Design review of the part built by this model. Coordinates are the model's own, in mm. Coordinates: 2 decimals unless noted, no trailing zeros. Write each loop counter-clockwise with the first axis right and the second up, starting at its lowest first coordinate (ties: lowest second). Pieces come first, ordered by that corner, then holes. Notation, with made-up numbers: (-2.75, 87.25) - (22.25, 87.25) arc R16 cw to (22.25, 93.25) - close; hole circle Ø2 at (-14.75, 70.25). An arc over 180 degrees is marked (long way). Use a Markdown table: item, result.
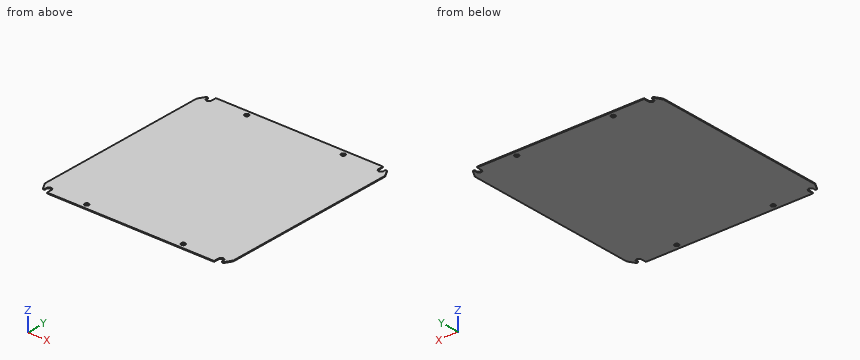
Autodesk Inventor part; units mm, degrees
ref_plane "DPF11_XY" through (224.5, 222.5, 0) normal (0, 0, 1) x (1, 0, 0)
ref_plane "DPF11_YZ" through (224.5, 222.5, 0) normal (1, 0, 0) x (0, 1, 0)
ref_plane "DPF11_ZX" through (224.5, 222.5, 0) normal (0, 1, 0) x (0, 0, 1)
sketch "Skizze_2" plane through (0, 0, 0) normal (0, 0, 1) x (1, 0, 0)
  line L0 (-224.5, 433.5455) -> (-224.5, 11.4545)
  line L1 (-224.5, 11.4545) -> (-215, -5)
  line L2 (-215, -5) -> (-211, -5)
  line L3 (-211, -5) -> (-211, 0)
  arc A0 (-199, 0) -> (-211, 0) centre (-205, 0) ccw
  line L4 (-199, 0) -> (-199, -12.5)
  line L5 (-199, -12.5) -> (199, -12.5)
  line L6 (199, -12.5) -> (199, 0)
  arc A1 (211, 0) -> (199, 0) centre (205, 0) ccw
  line L7 (211, 0) -> (211, -5)
  line L8 (211, -5) -> (215, -5)
  line L9 (215, -5) -> (224.5, 11.4545)
  line L10 (224.5, 11.4545) -> (224.5, 433.5455)
  line L11 (224.5, 433.5455) -> (215, 450)
  line L12 (215, 450) -> (211, 450)
  line L13 (211, 450) -> (211, 445)
  arc A2 (199, 445) -> (211, 445) centre (205, 445) ccw
  line L14 (199, 445) -> (199, 457.5)
  line L15 (199, 457.5) -> (-199, 457.5)
  line L16 (-199, 457.5) -> (-199, 445)
  arc A3 (-211, 445) -> (-199, 445) centre (-205, 445) ccw
  line L17 (-211, 445) -> (-211, 450)
  line L18 (-211, 450) -> (-215, 450)
  line L19 (-215, 450) -> (-224.5, 433.5455)
  circle A4 centre (115, 445) radius 5
  circle A5 centre (115, 0) radius 5
  circle A6 centre (-115, 445) radius 5
  circle A7 centre (-115, 0) radius 5
extrude "Extrusion1" add sketch "Skizze_2" against normal blind 2
ref_plane "DPF11_XY" through (224.5, 222.5, 0) normal (0, 0, 1) x (1, 0, 0)
ref_plane "DPF11_YZ" through (224.5, 222.5, 0) normal (1, 0, 0) x (0, 1, 0)
ref_plane "DPF11_ZX" through (224.5, 222.5, 0) normal (0, 1, 0) x (0, 0, 1)
ref_plane "DPF12_XY" through (-224.5, 222.5, 0) normal (0, 0, 1) x (1, 0, 0)
ref_plane "DPF12_YZ" through (-224.5, 222.5, 0) normal (1, 0, 0) x (0, 1, 0)
ref_plane "DPF12_ZX" through (-224.5, 222.5, 0) normal (0, 1, 0) x (0, 0, 1)
ref_plane "DPF21_XY" through (205, 445, 0) normal (0, 0, 1) x (1, 0, 0)
ref_plane "DPF21_YZ" through (205, 445, 0) normal (1, 0, 0) x (0, 1, 0)
ref_plane "DPF21_ZX" through (205, 445, 0) normal (0, 1, 0) x (0, 0, 1)
ref_plane "DPF22_XY" through (-205, 445, 0) normal (0, 0, 1) x (1, 0, 0)
ref_plane "DPF22_YZ" through (-205, 445, 0) normal (1, 0, 0) x (0, 1, 0)
ref_plane "DPF22_ZX" through (-205, 445, 0) normal (0, 1, 0) x (0, 0, 1)
ref_plane "DPG11_XY" through (0, -12.5, 0) normal (0, 0, 1) x (1, 0, 0)
ref_plane "DPG11_YZ" through (0, -12.5, 0) normal (1, 0, 0) x (0, 1, 0)
ref_plane "DPG11_ZX" through (0, -12.5, 0) normal (0, 1, 0) x (0, 0, 1)
ref_plane "DPG12_XY" through (0, 457.5, 0) normal (0, 0, 1) x (1, 0, 0)
ref_plane "DPG12_YZ" through (0, 457.5, 0) normal (1, 0, 0) x (0, 1, 0)
ref_plane "DPG12_ZX" through (0, 457.5, 0) normal (0, 1, 0) x (0, 0, 1)
ref_plane "DPG21_XY" through (205, 0, 0) normal (0, 0, 1) x (1, 0, 0)
ref_plane "DPG21_YZ" through (205, 0, 0) normal (1, 0, 0) x (0, 1, 0)
ref_plane "DPG21_ZX" through (205, 0, 0) normal (0, 1, 0) x (0, 0, 1)
ref_plane "DPG22_XY" through (205, 445, 0) normal (0, 0, 1) x (1, 0, 0)
ref_plane "DPG22_YZ" through (205, 445, 0) normal (1, 0, 0) x (0, 1, 0)
ref_plane "DPG22_ZX" through (205, 445, 0) normal (0, 1, 0) x (0, 0, 1)
ref_plane "montageplatte_XY" through (-205, 0, 0) normal (0, 0, 1) x (1, 0, 0)
ref_plane "montageplatte_YZ" through (-205, 0, 0) normal (1, 0, 0) x (0, 1, 0)
ref_plane "montageplatte_ZX" through (-205, 0, 0) normal (0, 1, 0) x (0, 0, 1)
properties part number "AE 1050_01_00 MontagePlatte"
(1) For L1, parallel to Y at x = 115, z = -0.95; L2, parallel to X at y = 445, z = -1.15, list the stretches that pass through material, from the lowest coordinate up. Write a range as from..to.
Determined:
| item | result |
|---|---|
| L1 | -12.5..-5, 5..440, 450..457.5 |
| L2 | -217.89..-211, -199..-120, -110..110, 120..199, 211..217.89 |
(2) Take a section at A-A on x = -205. Write out the cut boundary in (y, z), and give its area (3 significant figures).
Determined:
| item | result |
|---|---|
| outline | (6, -2) - (439, -2) - (439, 0) - (6, 0) - close |
| area | 866 mm2 |
(3) For pin 1 (0.6 mm diameter, centred on y = 449.5, z = -0.5, fed in from +X); pin 2 (1 mm diameter, centred on y = 446.5, z = -1.5, fed in from -X); pin 3 (10 mm diameter, centred on x = -105.5, y = 385.5, fed in from +Z); pin 4 (0.6 mm diameter, centred on x = 213, z = -1.5, fed in from -Y), all flat-tipped, find the tip position at first contact; note any pin that passes through.
Determined:
| item | result |
|---|---|
| pin 1 | x = 215.46 |
| pin 2 | x = -217.31 |
| pin 3 | z = 0 |
| pin 4 | y = -5 |
